from build123d import *

# Parameters (mm, degrees)
EXTRUDE_1_DEPTH = 8
CHAMFER_1_SIZE  = 4
CHAMFER_1_SIZE2 = 6.831877942
CHAMFER_2_SIZE  = 15
CHAMFER_2_SIZE2 = 9.944050138


with BuildPart() as part:
    # Эскиз1 → Вытянуть1 (new body)
    with BuildSketch(Plane.XY):
        Polygon((0, 0), (0, -26), (36, 0), align=None)
    extrude(amount=EXTRUDE_1_DEPTH)

    # Фаска1
    chamfer_1_edges = [part.edges().sort_by_distance(p)[0] for p in [
        (0, -26, 4),
    ]]
    chamfer_1_side = [part.faces().sort_by_distance(p)[0] for p in [
        (0, -13, 4),
    ]]
    chamfer(chamfer_1_edges, length=CHAMFER_1_SIZE, length2=CHAMFER_1_SIZE2, reference=chamfer_1_side[0])

    # Фаска2
    chamfer_2_edges = [part.edges().sort_by_distance(p)[0] for p in [
        (36, 0, 4),
    ]]
    chamfer_2_side = [part.faces().sort_by_distance(p)[0] for p in [
        (20.769230769, -11, 4),
    ]]
    chamfer(chamfer_2_edges, length=CHAMFER_2_SIZE, length2=CHAMFER_2_SIZE2, reference=chamfer_2_side[0])


solid = part.part
Model file for the job. Use its own axes, mm. Coordinates: 2 decimals unless noted, no trailing zeros. Write each loop counter-clockwise with the first axis right and the second up, starting at its lowest first coordinate (ties: lowest second). Pieces come first, ordered by that corner, then holes. Notation, with made-up numbers: (-25, 38) -> (3, 38) arc R19 cw to (3, 70) -> close; hole circle Ø3 at (55, 56). An arc over 180 degrees is marked (long way). One line per item, written item: value. Start each with the question number.
1) Slice it at A-A on z = 7. Write the cut outline in (x, y), then the cut area to 3 significant figures.
2) Slice it at C-C on y = -14.5. Write the cut outline in (x, z), then the cut area to 3 significant figures.
3) Slice it at B-B on x = 8.75. Write the cut outline in (y, z), then the cut area to 3 significant figures.
4) Flat gauge pins, fed straight in: pin 1 Ø2 at (x, z) = (22.5, 1.5) entering from -Y; pin 2 Ø2 at (y, z) = (-14.5, 6) entering from +X; pin 3 Ø1.5 at (y, z) = (-5, 1) entering from +X. Where does each tip first touch, or does it go through?
5) Probe probe 1 along X at (y, z) = (-10.75, 1.25); probe 2 along X at (y, z) = (-9.75, 5.75); probe 3 along Y at (x, z) = (12.5, 6.75). List the from-to ranges inside material, lowest first.
Answers follow:
1. outline: (0, -22) -> (5.54, -22) -> (23.84, -8.78) -> (26.06, 0) -> (0, 0) -> close
1. area: 413 mm2
2. outline: (0, 0) -> (15.92, 0) -> (15.92, 8) -> (0, 8) -> close
2. area: 127 mm2
3. outline: (-19.68, 0) -> (0, 0) -> (0, 8) -> (-19.68, 8) -> close
3. area: 157 mm2
4. pin 1: y = -10.47
4. pin 2: x = 17.31
4. pin 3: x = 24.98
5. probe 1: 0 to 21.12
5. probe 2: 0 to 22.5
5. probe 3: -16.97 to 0
